Check sheet for the modelled part. Datum: model origin and axes. Units: mm. A direction names the side the tool comes from. Round coordinates to 2 decimals unless told otherwise and drop trailing zeros.
Item 1: Go/stop test with flat-tipped pins: pin 1 Ø2 at (x, z) = (2.5, -40) entering from +Y; pin 2 Ø3 at (x, z) = (2.5, -40) entering from +Y. Record where each tip stops, or that it passes through.
Item 2: Material ranges on line 1 (Z direction, x = 2.5, y = 62.25); line 2 (X direction, y = 63, z = -40); line 3 (Z direction, x = 3.05, y = 57.5), recorded low to high.
Item 3: Tool access check on faces 1 (the flat face through (2, 0, -23)), 2 (the cylindrical face through (4.12, 3.55, -5.51)), 3 (the cylindrical face through (1.7, 61.5, -38.5)). Record the directions out of +Z, -Z, +X, -X, +Y, -Y that give a thin tool (end or side, any length) a straight path to the whole face; none if there is none.
Item 4: Release check for a two-part mould opening along Z. For faces 4 (the cylindrical face through (1.7, 61.5, -3.5)), 5 (the flat face through (2, 32, 0)), 6 (the flat face through (2, 32, -45)) record: +Z half, -Z half, draft (parallel to the pull), parting line (faces both ways), or undercut.
from build123d import *

# Parameters (mm, degrees)
SKETCH1_W                = 5
SKETCH1_H                = 45
BOSS_EXTRUDE1_DEPTH      = 65
M3_CLEARANCE_HOLE1_D     = 3.4
M3_CLEARANCE_HOLE1_DEPTH = 7
M3_CLEARANCE_HOLE1_TIP   = 1.021463052
M3_CLEARANCE_HOLE2_D     = 3.4
M3_CLEARANCE_HOLE2_DEPTH = 7
M3_CLEARANCE_HOLE2_TIP   = 1.021463052


with BuildPart() as part:
    # Sketch1 → Boss-Extrude1 (new body)
    with BuildSketch(Plane(origin=(0, 0, 0), x_dir=(1, 0, 0), z_dir=(0, 1, 0))):
        with Locations((2.5, 22.5)):
            Rectangle(SKETCH1_W, SKETCH1_H)
    extrude(amount=BOSS_EXTRUDE1_DEPTH)

    # M3 Clearance Hole1
    with Locations(Plane(origin=(0, 65, 0), x_dir=(1, 0, 0), z_dir=(0, 1, 0))):
        with Locations((2.5, 40), (2.5, 5)):
            Hole(M3_CLEARANCE_HOLE1_D / 2, depth=M3_CLEARANCE_HOLE1_DEPTH)
            with Locations((0, 0, -(M3_CLEARANCE_HOLE1_DEPTH + M3_CLEARANCE_HOLE1_TIP / 2))):  # 118° drill point
                Cone(0, M3_CLEARANCE_HOLE1_D / 2, M3_CLEARANCE_HOLE1_TIP, mode=Mode.SUBTRACT)

    # M3 Clearance Hole2
    with Locations(Plane(origin=(0, 0, 0), x_dir=(-1, 0, 0), z_dir=(0, -1, 0))):
        with Locations((-2.5, 39.999655037), (-2.5, 4.999655037)):
            Hole(M3_CLEARANCE_HOLE2_D / 2, depth=M3_CLEARANCE_HOLE2_DEPTH)
            with Locations((0, 0, -(M3_CLEARANCE_HOLE2_DEPTH + M3_CLEARANCE_HOLE2_TIP / 2))):  # 118° drill point
                Cone(0, M3_CLEARANCE_HOLE2_D / 2, M3_CLEARANCE_HOLE2_TIP, mode=Mode.SUBTRACT)


solid = part.part
Response values:
1. pin 1: stops at y = 57.58
1. pin 2: stops at y = 57.88
2. line 1: z = -45 to -41.7, -38.3 to -6.7, -3.3 to 0
2. line 2: x = 0 to 0.8, 4.2 to 5
2. line 3: z = -45 to -40.67, -39.33 to -5.67, -4.33 to 0
3. face 1: +Z, -Z, +X, -X, -Y
3. face 2: -Y
3. face 3: +Y
4. face 4: undercut
4. face 5: +Z half
4. face 6: -Z half
